For this review, take the finished solid that the model builds, in its own axes (mm). Face numbers are marked on the shaded views. Round coordinates to 2 decimals unless told otherwise and drop trailing zeros. Write each loop counter-clockwise with the first axis right and the second up, starting at its lowest first coordinate (ties: lowest second). Pieces come first, ordered by that corner, then holes. Notation, with made-up numbers: (-28.5, -31.5) - (-15.5, -31.5) arc R18 cw to (-15.5, -27.5) - close; hole circle Ø2 at (-20.75, -13.75). An arc over 180 degrees is marked (long way). Answer in a Markdown table with one row per item. Add a question column.
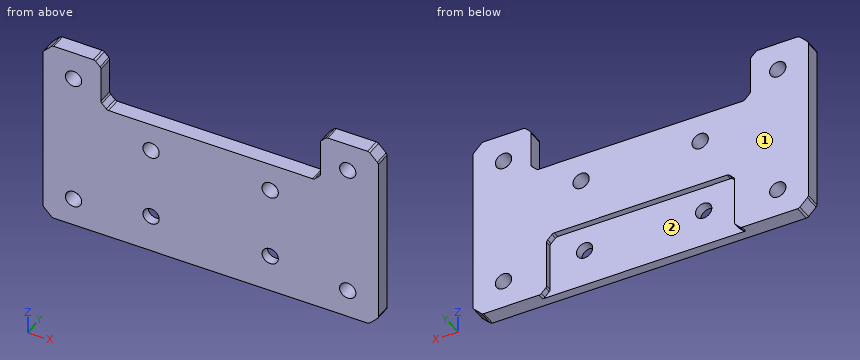
from build123d import *

# Parameters (mm, degrees)
SKETCH1_W                   = 107
SKETCH1_H                   = 60
BOSS_EXTRUDE1_DEPTH         = 5
SKETCH2_W                   = 60
SKETCH2_H                   = 20
CUT_EXTRUDE1_DEPTH          = 2
CUT_EXTRUDE2_REACH          = 7
SKETCH3_W                   = 70
SKETCH3_H                   = 16
CHAMFER1_SIZE               = 2
CHAMFER2_SIZE               = 3
FILLET1_R                   = 1
TAP_DRILL_FOR_M5_TAP1_D     = 5.2
TAP_DRILL_FOR_M5_TAP1_DEPTH = 46
TAP_DRILL_FOR_M5_TAP1_TIP   = 1.562237609
TAP_DRILL_FOR_M5_TAP2_D     = 5.2
TAP_DRILL_FOR_M5_TAP2_DEPTH = 46
TAP_DRILL_FOR_M5_TAP2_TIP   = 1.562237609


with BuildPart() as part:
    # Sketch1 → Boss-Extrude1 (new body)
    with BuildSketch(Plane(origin=(0, 0, 0), x_dir=(1, 0, 0), z_dir=(0, 1, 0))):
        Rectangle(SKETCH1_W, SKETCH1_H)
    extrude(amount=BOSS_EXTRUDE1_DEPTH)

    # Sketch2 → Cut-Extrude1 (cut)
    with BuildSketch(Plane(origin=(0, 5, 0), x_dir=(1, 0, 0), z_dir=(0, 1, 0))):
        with Locations((0, 20)):
            Rectangle(SKETCH2_W, SKETCH2_H)
    extrude(amount=-CUT_EXTRUDE1_DEPTH, mode=Mode.SUBTRACT)

    # Sketch3 → Cut-Extrude2 (cut, up to next)
    with BuildSketch(Plane(origin=(0, 5, 0), x_dir=(1, 0, 0), z_dir=(0, 1, 0)), mode=Mode.PRIVATE) as cut_extrude2_sk1:
        with Locations((0, -22)):
            Rectangle(SKETCH3_W, SKETCH3_H)
    cut_extrude2_tool1 = extrude(cut_extrude2_sk1.sketch, amount=-CUT_EXTRUDE2_REACH, mode=Mode.PRIVATE) & part.part
    add(cut_extrude2_tool1.solids().sort_by_distance((0, 5, 22))[0], mode=Mode.SUBTRACT)

    # Chamfer1
    chamfer1_edges = [part.edges().sort_by_distance(p)[0] for p in [
        (-30, 4, -10),
        (-30, 4, -30),
        (30, 4, -30),
        (30, 4, -10),
        (35, 2.5, 14),
        (35, 2.5, 30),
        (-35, 2.5, 30),
        (-35, 2.5, 14),
    ]]
    chamfer(chamfer1_edges, length=CHAMFER1_SIZE)

    # Chamfer2
    chamfer2_edges = [part.edges().sort_by_distance(p)[0] for p in [
        (53.5, 2.5, 30),
        (-53.5, 2.5, 30),
        (-53.5, 2.5, -30),
        (53.5, 2.5, -30),
    ]]
    chamfer(chamfer2_edges, length=CHAMFER2_SIZE)

    # Fillet1
    fillet1_edges = [part.edges().sort_by_distance(p)[0] for p in [
        (53.5, 2.5, -27),
        (53.5, 2.5, 27),
        (50.5, 2.5, 30),
        (-50.5, 2.5, -30),
        (50.5, 2.5, -30),
        (-53.5, 2.5, 27),
        (-53.5, 2.5, -27),
        (-50.5, 2.5, 30),
        (-32, 4, -30),
        (32, 4, -30),
        (30, 4, -12),
        (30, 4, -28),
        (-28, 4, -10),
        (28, 4, -10),
        (-30, 4, -28),
        (-30, 4, -12),
        (35, 2.5, 16),
        (35, 2.5, 28),
        (37, 2.5, 30),
        (-33, 2.5, 14),
        (33, 2.5, 14),
        (-35, 2.5, 28),
        (-35, 2.5, 16),
        (-37, 2.5, 30),
    ]]
    fillet(fillet1_edges, radius=FILLET1_R)

    # Tap Drill for M5 Tap1
    with Locations(Plane(origin=(-43.75, 5, -21), x_dir=(0, 0, 1), z_dir=(0, 1, 0))):
        with Locations((0, 0), (42, 0), (26, 24.75), (26, 62.75), (0, 87.5), (42, 87.5)):
            Hole(TAP_DRILL_FOR_M5_TAP1_D / 2, depth=TAP_DRILL_FOR_M5_TAP1_DEPTH)
            with Locations((0, 0, -(TAP_DRILL_FOR_M5_TAP1_DEPTH + TAP_DRILL_FOR_M5_TAP1_TIP / 2))):  # 118° drill point
                Cone(0, TAP_DRILL_FOR_M5_TAP1_D / 2, TAP_DRILL_FOR_M5_TAP1_TIP, mode=Mode.SUBTRACT)

    # Tap Drill for M5 Tap2
    with Locations(Plane(origin=(-19, 3, -18), x_dir=(0, 0, 1), z_dir=(0, 1, 0))):
        with Locations((0, 0), (0, 38)):
            Hole(TAP_DRILL_FOR_M5_TAP2_D / 2, depth=TAP_DRILL_FOR_M5_TAP2_DEPTH)
            with Locations((0, 0, -(TAP_DRILL_FOR_M5_TAP2_DEPTH + TAP_DRILL_FOR_M5_TAP2_TIP / 2))):  # 118° drill point
                Cone(0, TAP_DRILL_FOR_M5_TAP2_D / 2, TAP_DRILL_FOR_M5_TAP2_TIP, mode=Mode.SUBTRACT)


solid = part.part
Q1. Add section B-B on x = 43.75. State the section outline as (y, z) points, then the cut area to 3 significant figures.
Q2. To check wall thickness, follow probe 1 along X at (y, z) = (3.45, 5); probe 2 along X at (y, z) = (1.6, 20.5); probe 3 along X at (y, z) = (3.85, -16). State the ranges of each line that lie inside material, in increasing order.
Q3. Add section C-C on z = -13.5. State the section outline as (x, y) points.
Q4. Insertion check: pin 1 Ø16 at (x, z) = (-14.5, -22) entering from +Y; pin 2 Ø2 at (x, y) = (-36, 0.5) entering from +Z; pin 3 Ø2 at (x, y) = (7.5, 4) entering from +Z. Each pin has a flat end and moves straight along its axis. Give the tip position at first contact, or say it passes through.
Q5. Add section D-D on z = 4.5. State the section outline as (x, y) points, then the cut area to 3 significant figures.
Q6. Draft analysis for pull direction X (two halves, no side actions). For the marked faces 1 and 2, state which applies: released by +X, released by -X, zero draft, split by the parting line, or undercut.
Q7. Add section A-A on z = 21. State the section outline as (x, y) points, then the cut area to 3 significant figures.
Answer sheet:
| question | item | result |
|---|---|---|
| 1 | outline | (0, -30) - (5, -30) - (5, -23.6) - (0, -23.6) - close; (0, -18.4) - (5, -18.4) - (5, 18.4) - (0, 18.4) - close; (0, 23.6) - (5, 23.6) - (5, 30) - (0, 30) - close |
| 1 | area | 248 mm² |
| 2 | probe 1 | x = -53.5 to -21.6, -16.4 to 16.4, 21.6 to 53.5 |
| 2 | probe 2 | x = -53.5 to -46.3, -41.2 to -35, 35 to 41.2, 46.3 to 53.5 |
| 2 | probe 3 | x = -53.5 to -30, 30 to 53.5 |
| 3 | outline | (-53.5, 0) - (53.5, 0) - (53.5, 5) - (30, 5) - (30, 3) - (-30, 3) - (-30, 5) - (-53.5, 5) - close |
| 4 | pin 1 | stops at y = 3 |
| 4 | pin 2 | stops at z = 29.91 |
| 4 | pin 3 | stops at z = 14 |
| 5 | outline | (-53.5, 0) - (-21.55, 0) - (-21.55, 5) - (-53.5, 5) - close; (-16.45, 0) - (16.45, 0) - (16.45, 5) - (-16.45, 5) - close; (21.55, 0) - (53.5, 0) - (53.5, 5) - (21.55, 5) - close |
| 5 | area | 484 mm² |
| 6 | face 1 | zero draft |
| 6 | face 2 | undercut |
| 7 | outline | (-53.5, 0) - (-46.35, 0) - (-46.35, 5) - (-53.5, 5) - close; (-41.15, 0) - (-35, 0) - (-35, 5) - (-41.15, 5) - close; (35, 0) - (41.15, 0) - (41.15, 5) - (35, 5) - close; (46.35, 0) - (53.5, 0) - (53.5, 5) - (46.35, 5) - close |
| 7 | area | 133 mm² |
